Build history of the part. All positions in model axes, mm. Face numbers are marked on the shaded views. A direction names the side the tool comes from. Give positions to 0.01 mm unless a question says otherwise; leave off trailing zeros. Order: outer loops, then holes, each group sorted by start corner. A loop starts at its lowest first (then second) coordinate and runs counter-clockwise, first axis right, second up. Notation, with made-up numbers: (33.5, 44) - (75.5, 44) arc R6 cw to (75.5, 48) - close; hole circle Ø7 at (-12, 3). An arc over 180 degrees is marked (long way). Write each question's results on one line, items separated by ' | '. Start each with the question number.
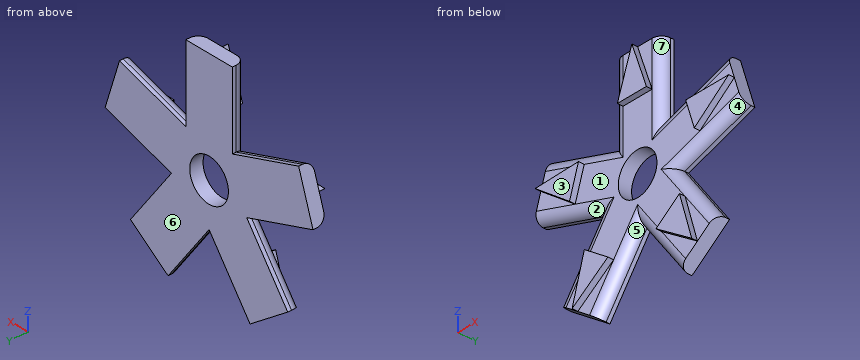
from build123d import *

# Parameters (mm, degrees)
F0_W     = 26.6942243119
F0_H     = 40
F1_DEPTH = 7
F2_R     = 5
F4_DEPTH = 3
F6_D     = 22.2
F6_DEPTH = 20
F6_TIP   = 6.6695528712


with BuildPart() as f1:
    # F0 (on Front) → F1 (new body)
    with BuildSketch(Plane.XZ):
        Polygon((-23.5114100917, -55.0681432643), (0, -22.7074634893), (-21.59608112, -7.0169921173), (-45.1074912117, -39.3776718923), align=None)
        Polygon((-21.59608112, -7.0169921173), (0, -22.7074634893), (21.59608112, -7.0169921173), (13.347112156, 18.370723862), (-13.347112156, 18.370723862), align=None)
        Polygon((21.59608112, -7.0169921173), (0, -22.7074634893), (23.5114100917, -55.0681432643), (45.1074912117, -39.3776718923), align=None)
        Polygon((-59.6383417718, 5.3436876577), (-21.59608112, -7.0169921173), (-13.347112156, 18.370723862), (-51.3893728078, 30.731403637), align=None)
        Polygon((13.347112156, 18.370723862), (21.59608112, -7.0169921173), (59.6383417718, 5.3436876577), (51.3893728078, 30.731403637), align=None)
        with Locations((0, 38.370723862)):
            Rectangle(F0_W, F0_H)
    extrude(amount=F1_DEPTH)

    # F2
    f2_edges = [f1.edges().sort_by_distance(p)[0] for p in [
        (-40.617211, -7, -0.836652),
        (-32.368242, -7, 24.551064),
        (-11.755705, -7, -38.887803),
        (40.617211, -7, -0.836652),
        (-33.351786, -7, -23.197332),
        (33.351786, -7, -23.197332),
        (11.755705, -7, -38.887803),
        (32.368242, -7, 24.551064),
        (13.347112, -7, 38.370724),
        (-13.347112, -7, 38.370724),
    ]]
    fillet(f2_edges, radius=F2_R)

    # F3 (on face) → F4 (join)
    with BuildSketch(Plane.XZ.offset(7)):
        Polygon((-55.5138572898, 18.0375456473), (-35.7995839881, 2.8553168412), (-30.6407849678, 18.7324676575), align=None)
        Polygon((0, 58.370723862), (-8.347112156, 34.9297690608), (8.347112156, 34.9297690608), align=None)
        Polygon((55.5138572898, 18.0375456473), (30.8665788163, 18.0375456473), (35.7995839881, 2.8553168412), align=None)
        Polygon((27.284158708, -23.3524673553), (13.7782475318, -33.1650862043), (34.3094506517, -47.2229075783), align=None)
        Polygon((-13.7782475318, -33.1650862043), (-27.284158708, -23.3524673553), (-34.3094506517, -47.2229075783), align=None)
    extrude(amount=F4_DEPTH)

    # F6
    with Locations(Plane(origin=(0, 0, 0), x_dir=(1, 0, 0), z_dir=(0, 1, 0))):
        with Locations((0, 0)):
            Hole(F6_D / 2, depth=F6_DEPTH)
            with Locations((0, 0, -(F6_DEPTH + F6_TIP / 2))):  # 118° drill point
                Cone(0, F6_D / 2, F6_TIP, mode=Mode.SUBTRACT)


solid = f1.part
Item 1: Cut at B-B, the plane z = 20.5. Count the separate pieces of the cut face and the enclosed holes in it, then the cut area to 3 significant figures.
Item 2: Flat gauge pins, fed straight in: pin 1 Ø0.9 at (x, y) = (44.5, -8) entering from +Z; pin 2 Ø9.5 at (x, z) = (-23.5, -46) entering from -Y; pin 3 Ø1.5 at (x, y) = (-23, -1) entering from +Z. Where does each tip first touch, or does it go through?
Item 3: Cut at A-A, the plane y = -5.5. List the corners of the cut face in (x, z).
Item 4: Which spindle directions (+Z, -Z, +X, -X, +Y, -Y) get a long thin tool onto all of the face, cutting with end or side? Do the marked faces 5, 6 and 7. Say none if no direction does.
Item 5: Probe line 1 along X through (y, z) = (-4, -43.5); line 2 along Y through (x, z) = (17, -3.5); line 3 along X through (y, z) = (-8, 9). List the from-to ranges inside material, lowest first. Write a range as from..to.
Item 6: Two-plate mould, pull along X, no slides. Class the marked faces 1, 2, 3 and 4: +X half, -X half, draft (parallel to the pull), parting line (faces both ways), or undercut.
Values found:
1) separate pieces: 3 | enclosed holes: 0 | area: 629 mm2
2) pin 1: stops at z = 18.04 | pin 2: stops at y = -7 | pin 3: stops at z = 21.75
3) outline: (-59.2, 6.7) - (-19.28, -6.27) - (-43.95, -40.22) - (-24.67, -54.23) - (0, -20.28) - (24.67, -54.23) - (43.95, -40.22) - (19.28, -6.27) - (59.2, 6.7) - (51.83, 29.37) - (11.92, 16.4) - (11.92, 58.37) - (-11.92, 58.37) - (-11.92, 16.4) - (-51.83, 29.37) - close; hole circle Ø22.2 at (0, 0)
4) face 5: -Z, -Y | face 6: +Z, -Z, +X, -X, +Y | face 7: +Z, -Y
5) line 1: x = -39.43..-15.62, 15.62..39.43 | line 2: y = -6.99..0 | line 3: x = -43.78..-33.8, 33.8..43.78
6) face 1: undercut | face 2: -X half | face 3: draft | face 4: +X half
